```python
from build123d import *

# Parameters (mm, degrees)
ESBO_O1_R                  = 1.6
RESSALTO_EXTRUS_O1_DEPTH   = 6
ESBO_O5_R                  = 1.6
RESSALTO_EXTRUS_O2_DEPTH   = 6
ESBO_O2_R                  = 1.6
CORTE_EXTRUS_O1_DEPTH      = 1
CORTE_EXTRUS_O1_DEPTH_BACK = 10


with BuildPart() as part:
    # Esboço1 → Ressalto-extrusão1 (new body)
    with BuildSketch(Plane.XZ.offset(6)):
        with BuildLine():
            Line((23.658239146, -5.419790473), (1.830835365, 3.169198905))
            ThreePointArc((1.830835365, 3.169198905), (0, 3.516453278), (-1.830835365, 3.169198905))
            Line((-1.830835365, 3.169198905), (-23.658239146, -5.419790473))
            ThreePointArc((-23.658239146, -5.419790473), (-25.806836409, -7.98111819), (-24.825744035, -11.177104364))
            Line((-24.825744035, -11.177104364), (-20.101514858, -15.804403192))
            ThreePointArc((-20.101514858, -15.804403192), (-18.128320556, -16.683568025), (-16.059952818, -16.060445681))
            Line((-16.059952818, -16.060445681), (-6.643887712, -8.924606384))
            ThreePointArc((-6.643887712, -8.924606384), (0, -6.691518958), (6.643887712, -8.924606384))
            Line((6.643887712, -8.924606384), (16.059952818, -16.060445681))
            ThreePointArc((16.059952818, -16.060445681), (18.128320556, -16.683568025), (20.101514858, -15.804403192))
            Line((20.101514858, -15.804403192), (24.825744035, -11.177104364))
            ThreePointArc((24.825744035, -11.177104364), (25.806836409, -7.98111819), (23.658239146, -5.419790473))
        make_face()
        with Locations((-17.932321173, -13.589770319)):
            Circle(ESBO_O1_R, mode=Mode.SUBTRACT)
        Circle(ESBO_O1_R, mode=Mode.SUBTRACT)
        with Locations((17.932321173, -13.589770319)):
            Circle(ESBO_O1_R, mode=Mode.SUBTRACT)
        with Locations((-22.376654391, -8.676712411)):
            Circle(ESBO_O1_R, mode=Mode.SUBTRACT)
        with Locations((22.376654391, -8.676712411)):
            Circle(ESBO_O1_R, mode=Mode.SUBTRACT)
    extrude(amount=-RESSALTO_EXTRUS_O1_DEPTH)

    # Esboço5 → Ressalto-extrusão2 (add)
    with BuildSketch(Plane.XZ.offset(6)):
        with Locations((17.932321173, -13.589770319)):
            Circle(ESBO_O5_R)
        with Locations((22.376654391, -8.676712411)):
            Circle(ESBO_O5_R)
    extrude(amount=-RESSALTO_EXTRUS_O2_DEPTH)

    # Esboço2 → Corte-extrusão1 (cut, two sides)
    with BuildSketch(Plane.XZ.offset(6)) as corte_extrus_o1_sk:
        with BuildLine():
            Line((16.923117575, -10.30388989), (2.470733648, -6.972588263))
            ThreePointArc((2.470733648, -6.972588263), (4.660651706, -7.727668012), (6.643887712, -8.924606384))
            Line((6.643887712, -8.924606384), (16.059952818, -16.060445681))
            ThreePointArc((16.059952818, -16.060445681), (18.128320556, -16.683568025), (20.101514858, -15.804403192))
            Line((20.101514858, -15.804403192), (24.825744035, -11.177104364))
            ThreePointArc((24.825744035, -11.177104364), (25.806836409, -7.98111819), (23.658239146, -5.419790473))
            Line((23.658239146, -5.419790473), (19.005551183, -3.588977798))
            ThreePointArc((19.005551183, -3.588977798), (21.081563864, -7.913151406), (16.923117575, -10.30388989))
        make_face()
        with Locations((17.714851393, -6.869063992)):
            Circle(ESBO_O2_R)
    extrude(amount=CORTE_EXTRUS_O1_DEPTH, mode=Mode.SUBTRACT)
    extrude(corte_extrus_o1_sk.sketch, amount=-CORTE_EXTRUS_O1_DEPTH_BACK, mode=Mode.SUBTRACT)


solid = part.part
```
Model file for the job. Use its own axes, mm. A direction names the side the tool comes from. Give positions to 0.01 mm unless a question says otherwise; leave off trailing zeros. Order: outer loops, then holes, each group sorted by start corner. A loop starts at its lowest first (then second) coordinate and runs counter-clockwise, first axis right, second up.
1) Pin check, flat tips, straight feed: pin 1 (2.5 mm diameter, centred on x = 17.71, z = -6.87, fed in from -Y); pin 2 (1.5 mm diameter, centred on x = 2, y = -1, fed in from -Z). Stop position of each tip, or through.
2) Mould opens along X. For faces 3 (the flat face through (-12.592, -3.042, -1.065)), 4 (the cylindrical face through (-1.27, -3.04, -0.97)), 5 (the flat face through (-3, -6, -4)) say: +X half, -X half, draft (parallel to the pull), parting line (faces both ways), or undercut.
3) Saw through at A-A, the plane x = 0. Write the cut outline in (y, z).
4) Saw through at B-B, the plane z = 0. Write the cut outline in (x, y).
5) 3-axis set-ups, long thin cutter, end or side, ignore diameter. For faces 1 (the flat face through (-3, 0, -4)), 2 (the flat face through (-11.418, -3.042, -12.542)): which of +Z, -Z, +X, -X, +Y, -Y reach the whole face in a straight line?
6) Saw through at D-D, the plane y = -2.7. Write the cut outline in (x, z), then the cut area to 3 significant figures.
7) Wall check: probe 1 along Z at (x, y) = (0, -2.75); probe 2 along X at (y, z) = (-0.5, -13.75); probe 3 along Z at (x, y) = (-21.5, -2.3). Give the ranges that are in metal, low to high.
8) Saw through at C-C, the plane z = -8. Write the cut outline in (x, y).
Computed:
1. pin 1: passes through
1. pin 2: stops at z = -7.04
2. face 3: -X half
2. face 4: undercut
2. face 5: draft
3. outline: (-6, -6.69) - (0, -6.69) - (0, -1.6) - (-6, -1.6) - close; (-6, 1.6) - (0, 1.6) - (0, 3.52) - (-6, 3.52) - close
4. outline: (-9.88, -6) - (-1.6, -6) - (-1.6, 0) - (-9.88, 0) - close; (1.6, -6) - (9.88, -6) - (9.88, 0) - (1.6, 0) - close
5. face 1: +Z, -Z, +X, -X, +Y
5. face 2: -Z, +Y, -Y
6. outline: (-24.83, -11.18) - (-20.1, -15.8) arc R3.1 ccw to (-16.06, -16.06) - (-6.64, -8.92) arc R11 cw to (2.47, -6.97) - (16.92, -10.3) arc R3.52 ccw to (19.01, -3.59) - (1.83, 3.17) arc R5 ccw to (-1.83, 3.17) - (-23.66, -5.42) arc R3.5 ccw to start; hole circle Ø3.2 at (-22.38, -8.68); hole circle Ø3.2 at (-17.93, -13.59); hole circle Ø3.2 at (0, 0); hole circle Ø3.2 at (17.71, -6.87)
6. area: 420 mm2
7. probe 1: z = -6.69 to -1.6, 1.6 to 3.52
7. probe 2: x = -22.2 to -19.52, -16.34 to -13.01
7. probe 3: z = -14.43 to -10.02, -7.34 to -4.57
8. outline: (-25.81, -6) - (-23.83, -6) - (-23.83, 0) - (-25.81, 0) - close; (-20.93, -6) - (-5.2, -6) - (-5.2, 0) - (-20.93, 0) - close; (6.93, -6) - (16.58, -6) - (16.58, 0) - (6.93, 0) - close; (18.85, -6) - (21.05, -6) - (21.05, 0) - (18.85, 0) - close
